Here's the drawing with two shaded views (mm, measured from the low corner). I have some questions. A direction names the side the tool comes from. Coordinates: 2 decimals unless noted, no trailing zeros. Write each loop counter-clockwise with the first axis right and the second up, starting at its lowest first coordinate (ties: lowest second). Pieces come first, ordered by that corner, then holes.
Item 1: I want a section at C-C on x = 4. Please give me the cut outline in (y, z), then the cut area to 3 significant figures.
Item 2: I want a section at A-A on y = 38. Please give me the cut outline in (x, z).
Item 3: For P1, Ø1.5, axis at y = 38, z = 11, coming from the +X side; P2, Ø6, axis at x = 33, z = 38, coming from the -Y side; P3, Ø8.5, axis at y = 64.92, z = 38, coming from the -X side, each with a flat end and sliding along its axis, tell me the tip position at first contact or that it passes through.
Item 4: I want a section at B-B on z = 38. Please give me the cut outline in (x, y), then the cut area to 3 significant figures.
Item 5: I want a section at D-D on x = 32. Please give me the cut outline in (y, z), then the cut area to 3 significant figures.
Item 6: Thinking about a two-plate mould opening in Z: for the marked faces 3 and 4, which applies, +Z half, -Z half, draft (parallel to the pull), parting line (faces both ways), or undercut?
Item 7: If I drill on probe 1 along Y at (x, z) = (20, 38); probe 2 along Y at (x, z) = (22, 40); probe 3 along Z at (x, y) = (8, 27) (1 decimal), over which ranges is the centre line in solid material (lowest first)?
Item 8: Which directions (+Z, -Z, +X, -X, +Y, -Y) give clear straight access to the entire face, cutting with the end or side of a thin tool? Please do the marked faces 1 and 2.
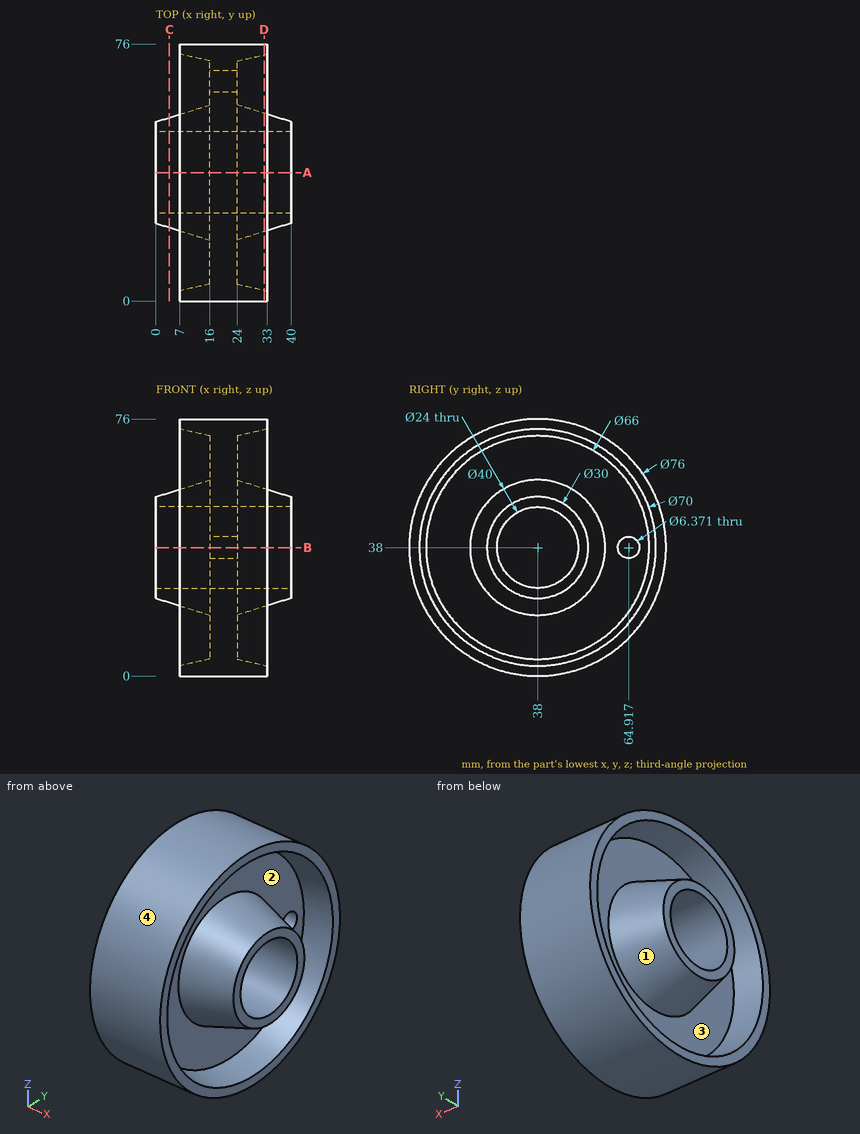
Response values:
1. outline: circle Ø32.5 at (38, 38); hole circle Ø24 at (38, 38)
1. area: 377 mm2
2. outline: (0, 23) - (16, 18) - (16, 5) - (7, 3) - (7, 0) - (33, 0) - (33, 3) - (24, 5) - (24, 18) - (40, 23) - (40, 26) - (0, 26) - close; (0, 50) - (40, 50) - (40, 53) - (24, 58) - (24, 71) - (33, 73) - (33, 76) - (7, 76) - (7, 73) - (16, 71) - (16, 58) - (0, 53) - close
3. P1: stops at x = 24
3. P2: stops at y = 0
3. P3: stops at x = 16
4. outline: (0, 23) - (16, 18) - (16, 5) - (7, 3) - (7, 0) - (33, 0) - (33, 3) - (24, 5) - (24, 18) - (40, 23) - (40, 26) - (0, 26) - close; (0, 50) - (40, 50) - (40, 53) - (24, 58) - (24, 61.73) - (16, 61.73) - (16, 58) - (0, 53) - close; (7, 73) - (16, 71) - (16, 68.1) - (24, 68.1) - (24, 71) - (33, 73) - (33, 76) - (7, 76) - close
4. area: 861 mm2
5. outline: circle Ø76 at (38, 38); circle Ø35 at (38, 38); hole circle Ø69.56 at (38, 38); hole circle Ø24 at (38, 38)
5. area: 1,250 mm2
6. face 3: undercut
6. face 4: parting line
7. probe 1: y = 0 to 26, 50 to 61.73, 68.1 to 76
7. probe 2: y = 0.05 to 26.17, 49.83 to 62.44, 67.4 to 75.95
7. probe 3: z = 1.6 to 5, 24.4 to 33.2, 42.8 to 51.6, 71 to 74.4
8. face 1: -X
8. face 2: +X
